```python
from build123d import *

# Parameters (mm, degrees)
F0_R      = 30
F0_R_2    = 15
F1_DEPTH  = 20
F3_R      = 7.5
F4_DEPTH  = 13
F5_R      = 5
F6_DEPTH  = 65.5
F8_R      = 7.5
F9_DEPTH  = 13
F12_R     = 7.5
F13_DEPTH = 13
F14_R     = 5
F15_DEPTH = 92
F16_R     = 7.5
F17_DEPTH = 13
F19_DEPTH = 15
F18_R     = 0.5
F20_DEPTH = 15
F21_DEPTH = 15
F22_DEPTH = 15


with BuildPart() as f1:
    # F0 (on Front) → F1 (new body, symmetric)
    with BuildSketch(Plane.XZ):
        Circle(F0_R)
        Circle(F0_R_2, mode=Mode.SUBTRACT)
    extrude(amount=F1_DEPTH, both=True)

    # F3 (on offset) → F4 (cut)
    with BuildSketch(Plane.XY.offset(30)):
        Circle(F3_R)
    extrude(amount=-F4_DEPTH, mode=Mode.SUBTRACT)

    # F5 (on offset) → F6 (cut)
    with BuildSketch(Plane.XY.offset(30)):
        Circle(F5_R)
    extrude(amount=-F6_DEPTH, mode=Mode.SUBTRACT)

    # F8 (on offset) → F9 (cut)
    with BuildSketch(Plane.XY.offset(-30)):
        Circle(F8_R)
    extrude(amount=F9_DEPTH, mode=Mode.SUBTRACT)

    # F12 (on offset) → F13 (cut)
    with BuildSketch(Plane.YZ.offset(30)):
        Circle(F12_R)
    extrude(amount=-F13_DEPTH, mode=Mode.SUBTRACT)

    # F14 (on offset) → F15 (cut)
    with BuildSketch(Plane.YZ.offset(30)):
        Circle(F14_R)
    extrude(amount=-F15_DEPTH, mode=Mode.SUBTRACT)

    # F16 (on offset) → F17 (cut)
    with BuildSketch(Plane.YZ.offset(-30)):
        Circle(F16_R)
    extrude(amount=F17_DEPTH, mode=Mode.SUBTRACT)

    # F18 (on Front) → F19 (cut, symmetric)
    with BuildSketch(Plane.XZ):
        with BuildLine():
            ThreePointArc((0, 15.5), (0.353553, 15.646447), (0.5, 16))
            ThreePointArc((0.5, 16), (-0.353553, 16.353553), (0, 15.5))
        make_face()
    extrude(amount=F19_DEPTH, both=True, mode=Mode.SUBTRACT)

    # F18 (on Front) → F20 (cut, symmetric)
    with BuildSketch(Plane.XZ):
        with Locations((16, 0)):
            Circle(F18_R)
    extrude(amount=F20_DEPTH, both=True, mode=Mode.SUBTRACT)

    # F18 (on Front) → F21 (cut, symmetric)
    with BuildSketch(Plane.XZ):
        with Locations((0, -16)):
            Circle(F18_R)
    extrude(amount=F21_DEPTH, both=True, mode=Mode.SUBTRACT)

    # F18 (on Front) → F22 (cut, symmetric)
    with BuildSketch(Plane.XZ):
        with Locations((-16, 0)):
            Circle(F18_R)
    extrude(amount=F22_DEPTH, both=True, mode=Mode.SUBTRACT)


solid = f1.part
```
Part model, mm, in its own coordinate system. A direction names the side the tool comes from. Give positions to 0.01 mm unless a question says otherwise; leave off trailing zeros. Order: outer loops, then holes, each group sorted by start corner. A loop starts at its lowest first (then second) coordinate and runs counter-clockwise, first axis right, second up. Notation, with made-up numbers: M 9,55 L 62,55 A36 ccw 62,91 Z; hole C -20,-7 d7. An arc over 180 degrees is marked long. Use a Markdown table: item, result. Add a question column.
(1) Mould opens along Y. For faces 1 (the face through (6, -20, 14)), 2 (the face through (23.591, -7.493, 0.33)), 3 (the face through (6, 20, 14)) say: +Y half, -Y half, draft (parallel to the pull), parting line (faces both ways), or undercut.
(2) Saw through at A-A, the plane z = -3. Give the cut face in (x, y), and give its area (3 significant figures).
(3) Probe line 1 along X through (y, z) = (-9, 0); line 2 along X through (y, z) = (-15, -11.5); line 3 along Z through (x, y) = (4, 12.5). List the from-to ranges inside material, lowest first. Write a range as [from, to].
(4) Saw through at C-C, the plane y = 13.5. Give the cut face in (x, z), and give its area (3 significant figures).
(5) Drop flat-ended pins along their axis: P1, Ø7.5, axis at y = 2.5, z = -1.5, coming from the -X side; P2, Ø1.5, axis at y = -5.5, z = 20, coming from the -X side; P3, Ø12, axis at y = 4, z = 11.5, coming from the -X side. Give the stop position or say it passes through.
(6) Saw through at D-D, the plane x = -11. Give the cut face in (y, z).
(7) Saw through at B-B, the plane x = -24. Give the cut face in (y, z), and give its area (3 significant figures).
(8) 3-axis set-ups, long thin cutter, end or side, ignore diameter. For faces 4 (the face through (-23.591, -7.493, 0.33)), 5 (the face through (17, 2, -5)), 6 (the face through (-7.493, 0.33, -23.592)), 7 (the face through (4.619, -1.915, 15.909)), 8 (the face through (-7.493, 0.33, 23.592)): which of +Z, -Z, +X, -X, +Y, -Y reach the whole face in a straight line?
Answer key:
| question | item | result |
|---|---|---|
| 1 | face 1 | -Y half |
| 1 | face 2 | undercut |
| 1 | face 3 | +Y half |
| 2 | outline | M -29.85,-20 L -14.7,-20 L -14.7,-4 L -17,-4 L -17,-6.87 L -29.85,-6.87 Z; M -29.85,6.87 L -17,6.87 L -17,4 L -14.7,4 L -14.7,20 L -29.85,20 Z; M 14.7,-20 L 29.85,-20 L 29.85,-6.87 L 17,-6.87 L 17,-4 L 14.7,-4 Z; M 14.7,4 L 17,4 L 17,6.87 L 29.85,6.87 L 29.85,20 L 14.7,20 Z |
| 2 | area | 822 mm^2 |
| 3 | line 1 | [-30, -16.5], [-15.5, -15], [15, 15.5], [16.5, 30] |
| 3 | line 2 | [-27.71, -9.63], [9.63, 27.71] |
| 3 | line 3 | [-29.73, -14.46], [14.46, 29.73] |
| 4 | outline | C 0,0 d60; hole C -16,0 d1; hole C 0,0 d30; hole C 0,-16 d1; hole M 0,15.5 A0.5 ccw 0.5,16 A0.5 ccw long Z; hole C 16,0 d1 |
| 4 | area | 2,120 mm^2 |
| 5 | P1 | x = -17 |
| 5 | P2 | x = -23.01 |
| 5 | P3 | x = -29.48 |
| 6 | outline | M -20,-27.91 L 20,-27.91 L 20,-10.2 L -20,-10.2 Z; M -20,10.2 L 20,10.2 L 20,27.91 L -20,27.91 Z |
| 7 | outline | M -20,-18 L 20,-18 L 20,18 L -20,18 Z; hole C 0,0 d15 |
| 7 | area | 1,260 mm^2 |
| 8 | face 4 | -X |
| 8 | face 5 | +X |
| 8 | face 6 | -Z |
| 8 | face 7 | +Z, -Z |
| 8 | face 8 | +Z |
